Geometry: final body of the model. Coordinates: model frame, mm. Face numbers are marked on the shaded views. Round coordinates to 2 decimals unless told otherwise and drop trailing zeros. Loops run counter-clockwise (first coordinate to the right, second up) from the corner with the lowest first, then second, coordinate; pieces in that order, holes last. Notation, with made-up numbers: (31.5, 14) - (85.5, 14) arc R20 ccw to (85.5, 52) - close; hole circle Ø9 at (-0.5, 81.25). An arc over 180 degrees is marked (long way). Answer in a Markdown table with one row per item. Add a question column.
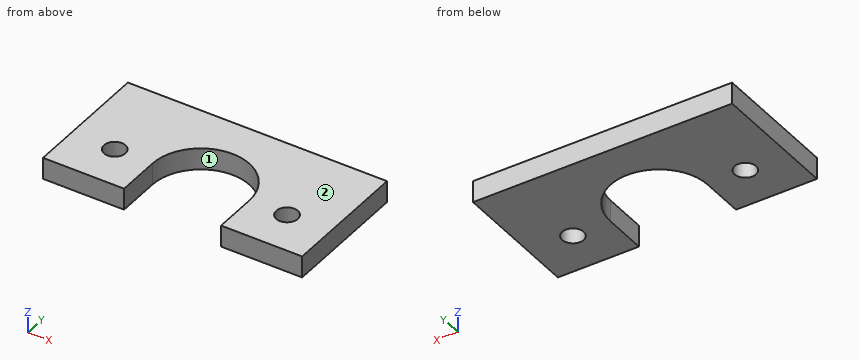
from build123d import *

# Parameters (mm, degrees)
SKETCH1_R           = 3.168199077
BOSS_EXTRUDE1_DEPTH = 6.35


with BuildPart() as part:
    # Sketch1 → Boss-Extrude1 (new body)
    with BuildSketch(Plane.XY):
        with BuildLine():
            Line((-14.256895846, 0.249783871), (-14.256895846, -12.450216129))
            Line((-14.256895846, -12.450216129), (-38.1, -12.450216129))
            Line((-38.1, -12.450216129), (-38.1, 25.649783871))
            Line((-38.1, 25.649783871), (38.1, 25.649783871))
            Line((38.1, 25.649783871), (38.1, -12.450216129))
            Line((38.1, -12.450216129), (14.256895846, -12.450216129))
            Line((14.256895846, -12.450216129), (14.256895846, 0.249783871))
            ThreePointArc((14.256895846, 0.249783871), (0, 14.506679717), (-14.256895846, 0.249783871))
        make_face()
        with Locations((-25.345592616, 0.249783871)):
            Circle(SKETCH1_R, mode=Mode.SUBTRACT)
        with Locations((25.345592616, 0.249783871)):
            Circle(SKETCH1_R, mode=Mode.SUBTRACT)
    extrude(amount=BOSS_EXTRUDE1_DEPTH)


solid = part.part
1) Pull-direction query (X, two-part tool) for the marked faces 1 and 2; classes: pulls with the +X half, pulls with the -X half, needs draft (parallel to the pull), parting line crosses it, or undercut.
2) Section C-C, the plane x = 0. Return the cut outline in (y, z).
3) Material intervals for line 1 along X through (y, z) = (0.5, 0.5); line 2 along X through (y, z) = (2.5, 1); line 3 along Y through (x, z) = (28, 1.75), sorted ascending. Write a range as from..to.
4) Section A-A, the plane y = -9.5. Return the cut outline in (x, z), and give its area (3 significant figures).
5) Section B-B, the plane z = 1.5. Return the cut outline in (x, y), and give its area (3 significant figures).
6) Section D-D, the plane x = 9.5. Return the cut outline in (y, z).
Evaluation:
| question | item | result |
|---|---|---|
| 1 | face 1 | undercut |
| 1 | face 2 | needs draft |
| 2 | outline | (14.51, 0) - (25.65, 0) - (25.65, 6.35) - (14.51, 6.35) - close |
| 3 | line 1 | x = -38.1..-28.5, -22.19..-14.25, 14.25..22.19, 28.5..38.1 |
| 3 | line 2 | x = -38.1..-27.58, -23.12..-14.08, 14.08..23.12, 27.58..38.1 |
| 3 | line 3 | y = -12.45..-1.48, 1.98..25.65 |
| 4 | outline | (-38.1, 0) - (-14.26, 0) - (-14.26, 6.35) - (-38.1, 6.35) - close; (14.26, 0) - (38.1, 0) - (38.1, 6.35) - (14.26, 6.35) - close |
| 4 | area | 303 mm² |
| 5 | outline | (-38.1, -12.45) - (-14.26, -12.45) - (-14.26, 0.25) arc R14.26 cw to (14.26, 0.25) - (14.26, -12.45) - (38.1, -12.45) - (38.1, 25.65) - (-38.1, 25.65) - close; hole circle Ø6.34 at (-25.35, 0.25); hole circle Ø6.34 at (25.35, 0.25) |
| 5 | area | 2,160 mm² |
| 6 | outline | (10.88, 0) - (25.65, 0) - (25.65, 6.35) - (10.88, 6.35) - close |
